Autodesk Inventor part; units mm, degrees
ref_plane "YZ Plane" through (0, 0, 0) normal (1, 0, 0) x (0, 1, 0)
ref_plane "XZ Plane" through (0, 0, 0) normal (0, 1, 0) x (-1, 0, 0)
ref_plane "XY Plane" through (0, 0, 0) normal (0, 0, 1) x (1, 0, 0)
sketch "Sketch1" plane through (0, 0, 0) normal (0, 0, 1) x (1, 0, 0)
  line L0 (0, 0) -> (12, 0)
  line L1 (12, 0) -> (12, 12)
  line L2 (12, 12) -> (0, 12)
  line L3 (0, 12) -> (0, 0)
  dimension "d0" = 12
  dimension "d1" = 12
extrude "Extrusion1" add sketch "Sketch1" along normal blind 4
fillet "Fillet1" radius 1 1 edges at (12, 12, 2)
fillet "Fillet2" radius 1 3 edges at (0, 12, 2) (12, 0, 2) (0, 0, 2)
sketch "Sketch2" plane through (0, 0, 4) normal (0, 0, 1) x (1, 0, 0)
  line L0 (1, 1) -> (11, 1)
  line L1 (11, 1) -> (11, 11)
  line L2 (11, 11) -> (1, 11)
  line L3 (1, 11) -> (1, 1)
  point P0 (0, 0)
  point P1 (1, 0)
  dimension "d7" = 1
  dimension "d8" = 10
  dimension "d9" = 10
extrude "Extrusion2" cut sketch "Sketch2" against normal blind 1
sketch "Sketch3" plane through (0, 0, 3) normal (0, 0, 1) x (1, 0, 0)
  point P0 (0, 0)
properties part number "BTN_1"
For this review, take the finished solid that the model builds, in its own axes (mm). A direction names the side the tool comes from. Round coordinates to 2 decimals unless told otherwise and drop trailing zeros. Write each loop counter-clockwise with the first axis right and the second up, starting at its lowest first coordinate (ties: lowest second). Pieces come first, ordered by that corner, then holes.
1) Machinability: for faces 1 (the face through (12, 6, 2)), 2 (the face through (1, 6.1, 3.5)), which of the approach directions +Z, -Z, +X, -X, +Y, -Y give a long, thin tool a straight path to every point of the face, cutting with its end or side? Answer none if there is none.
Answer below:
face 1: +Z, -Z, +X, +Y, -Y
face 2: +Z
2) Mouldability with a two-part tool opening along Y and no side actions: class faces 3 (the face through (0, 6, 2)), 4 (the face through (11.699, 0.285, 2.028)), 5 (the face through (6, 6, 3)) as +Y half, -Y half, draft (parallel to the pull), parting line (faces both ways), or undercut.
Answer below:
face 3: draft
face 4: -Y half
face 5: undercut
3) For line 1 along X through (y, z) = (6, 3.8); line 2 along Z through (x, y) = (6.5, 3), list the stretches that pass through material, from the lowest coordinate up.
Answer below:
line 1: x = 0 to 1, 11 to 12
line 2: z = 0 to 3
4) Take a section at A-A on z = 3.2. Give the boundary of the cut face in (x, y).
Answer below:
outline: (0, 1) arc R1 ccw to (1, 0) - (11, 0) arc R1 ccw to (12, 1) - (12, 11) arc R1 ccw to (11, 12) - (1, 12) arc R1 ccw to (0, 11) - close; hole (1, 1) - (11, 1) - (11, 11) - (1, 11) - close
5) Take a section at B-B on y = 8.5. Give the boundary of the cut face in (x, z), then the cut area to 3 significant figures.
Answer below:
outline: (0, 0) - (12, 0) - (12, 4) - (11, 4) - (11, 3) - (1, 3) - (1, 4) - (0, 4) - close
area: 38.0 mm2
